Answer from the drawing. Dimensions are ordinates in mm from the lowest x, y and z of the part. A direction names the side the tool comes from. Give positions to 0.01 mm unless a question says otherwise; leave off trailing zeros. Write each question's results on one line, items separated by ' | '.
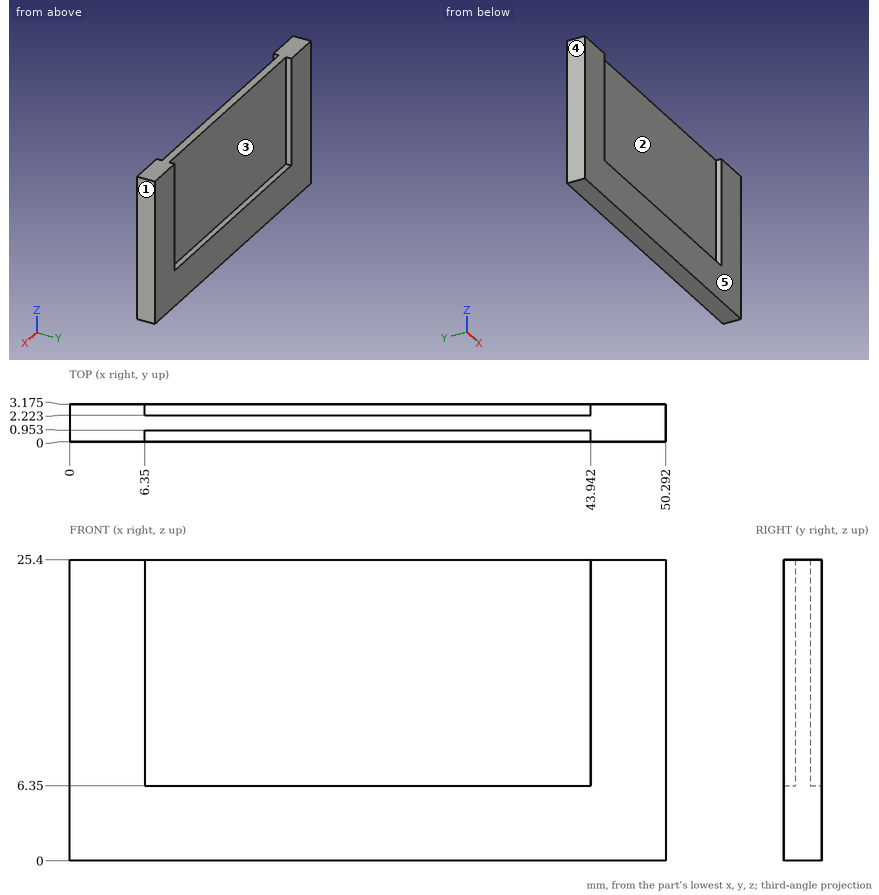
(1) The mould has two halves that part along X. Classify the marked faces 3, 4 and 5: pulls with the +X half, pulls with the -X half, needs draft (parallel to the pull), parting line crosses it, or undercut.
Conclusion:
face 3: undercut | face 4: pulls with the -X half | face 5: needs draft
(2) Each of these flat-tipped pins is pushed along its axis until it touches: pin 1 (1.5 mm diameter, centred on x = 23.5, y = 0.5, fed in from -Z); pin 2 (2 mm diameter, centred on x = 42.5, z = 13.5, fed in from +Y); pin 3 (0.5 mm diameter, centred on x = 25.5, y = 0.5, fed in from +Z); pin 4 (9.5 mm diameter, centred on x = 28, z = 12.5, fed in from -Y). Where does it stop, or does it pass through?
Conclusion:
pin 1: z = 0 | pin 2: y = 2.22 | pin 3: z = 6.35 | pin 4: y = 0.95
(3) For the marked faces 1 and 2, determine the directions among +Z, -Z, +X, -X, +Y, -Y from which every point of the face is accessible in a straight line to the end or side of a thin tool.
Conclusion:
face 1: +Z, -Z, +X, +Y, -Y | face 2: +Z, -Y
(4) Consider probe 1 along X at (y, z) = (2.95, 22); probe 2 along Y at (x, z) = (28, 21.5); probe 3 along Z at (x, y) = (36, 2.8). Determine where each line is inside the solid, lowest interval first. Write a range as [from, to].
Conclusion:
probe 1: [0, 6.35], [43.94, 50.29] | probe 2: [0.95, 2.22] | probe 3: [0, 6.35]
